Here's the drawing with two shaded views (mm, measured from the low corner). I have some questions. A direction names the side the tool comes from. Give positions to 0.01 mm unless a question says otherwise; leave off trailing zeros. Write each loop counter-clockwise with the first axis right and the second up, starting at its lowest first coordinate (ties: lowest second). Pieces come first, ordered by that corner, then holes. Notation, with made-up numbers: (82.5, -32.5) -> (117.5, -32.5) arc R17 cw to (117.5, -7.5) -> close; hole circle Ø8 at (46.5, 36). An arc over 180 degrees is marked (long way). One line per question, with ' | ' between items.
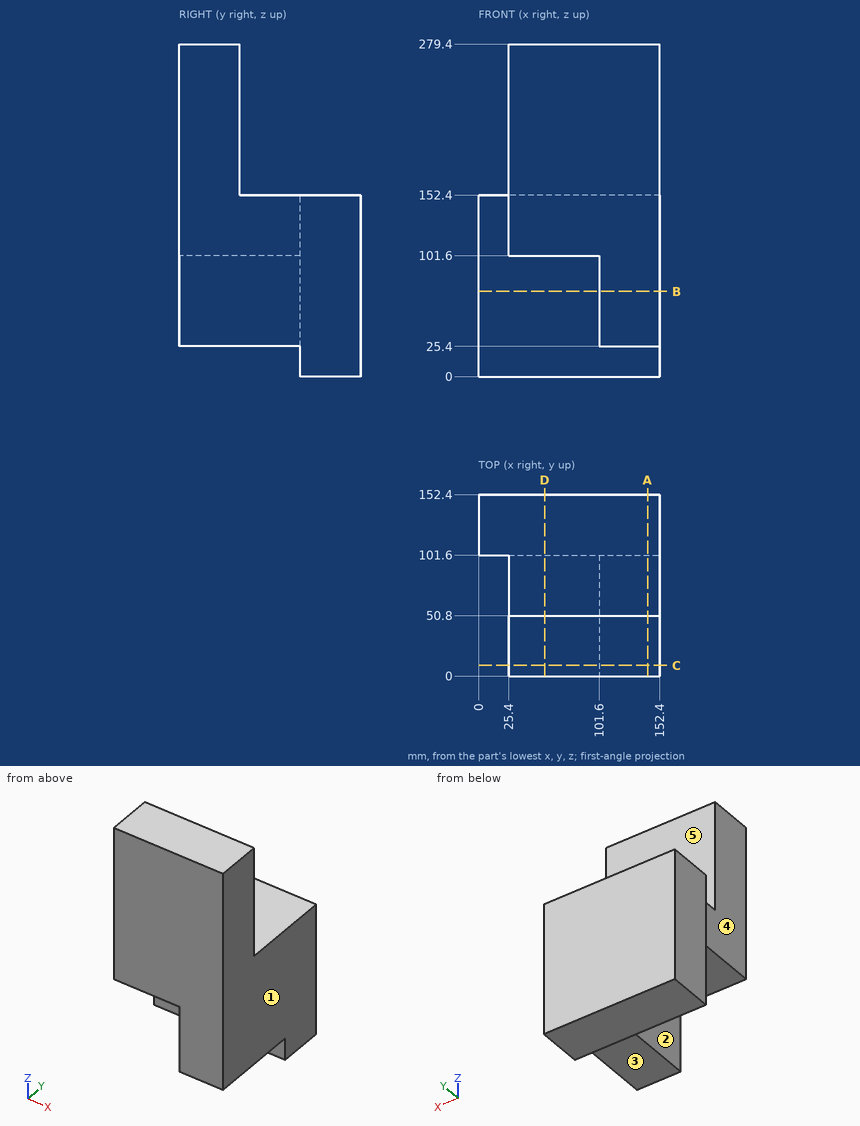
Q1. On a 3-axis mill with a long thin cutter (end or side, diameter ignored), from which of +Z, -Z, +X, -X, +Y, -Y can I reach the whole of each face in a straight line? I mean the marked faces 1, 2, 3, 4 and 5. Say none if no direction works.
Answer below:
face 1: +Z, -Z, +X, +Y, -Y | face 2: -Z, -X, -Y | face 3: -Z, +X, -X, -Y | face 4: +Z, -Z, -X, -Y | face 5: +Z, +X, -X, +Y
Q2. Imagine slicing it at B-B on z = 71.5. Please give me the cut outline in (x, y).
Answer below:
outline: (0, 101.6) -> (101.6, 101.6) -> (101.6, 0) -> (152.4, 0) -> (152.4, 152.4) -> (0, 152.4) -> close
Q3. Imagine slicing it at D-D on x = 55.5. Please give me the cut outline in (y, z).
Answer below:
outline: (0, 101.6) -> (101.6, 101.6) -> (101.6, 0) -> (152.4, 0) -> (152.4, 152.4) -> (50.8, 152.4) -> (50.8, 279.4) -> (0, 279.4) -> close
Q4. Imagine slicing it at C-C on y = 9. Please give me the cut outline in (x, z).
Answer below:
outline: (25.4, 101.6) -> (101.6, 101.6) -> (101.6, 25.4) -> (152.4, 25.4) -> (152.4, 279.4) -> (25.4, 279.4) -> close
Q5. Will these pins go through, and if not, where does the flat tip stop? pin 1 (6 mm diameter, centred on y = 119, z = 81.5, fed in from -X); pin 2 (23 mm diameter, centred on y = 66.5, z = 48.5, fed in from -X); pin 3 (23 mm diameter, centred on x = 58.5, y = 56.5, fed in from -Z); pin 4 (10 mm diameter, centred on x = 31, z = 53.5, fed in from -Y).
Answer below:
pin 1: stops at x = 0 | pin 2: stops at x = 101.6 | pin 3: stops at z = 101.6 | pin 4: stops at y = 101.6
Q6. If I drill on line 1 along X through (y, z) = (23, 246.5); line 2 along Z through (x, y) = (65.5, 101.5), over which ranges is the centre line in solid material (lowest first)?
Answer below:
line 1: x = 25.4 to 152.4 | line 2: z = 101.6 to 152.4
Q7. Imagine slicing it at A-A on x = 142. Please give me the cut outline in (y, z), and give its area (3 significant figures).
Answer below:
outline: (0, 25.4) -> (101.6, 25.4) -> (101.6, 0) -> (152.4, 0) -> (152.4, 152.4) -> (50.8, 152.4) -> (50.8, 279.4) -> (0, 279.4) -> close | area: 27,100 mm^2
